Input: dimensioned drawing with shaded views. Units: mm. Origin: part minimum x, y, z. A direction names the side the tool comes from. Give positions to 0.01 mm unless a question says otherwise; leave off trailing zeros. Write each loop counter-clockwise with the first axis right and the second up, starting at its lowest first coordinate (ties: lowest second). Pieces come first, ordered by that corner, then holes. Notation, with made-up numbers: (28.25, 22.5) -> (54.25, 22.5) arc R6 cw to (54.25, 26.5) -> close; hole circle Ø4 at (-39, 55). An arc over 180 degrees is marked (long way). Answer as a JSON object with one key per item and string values.
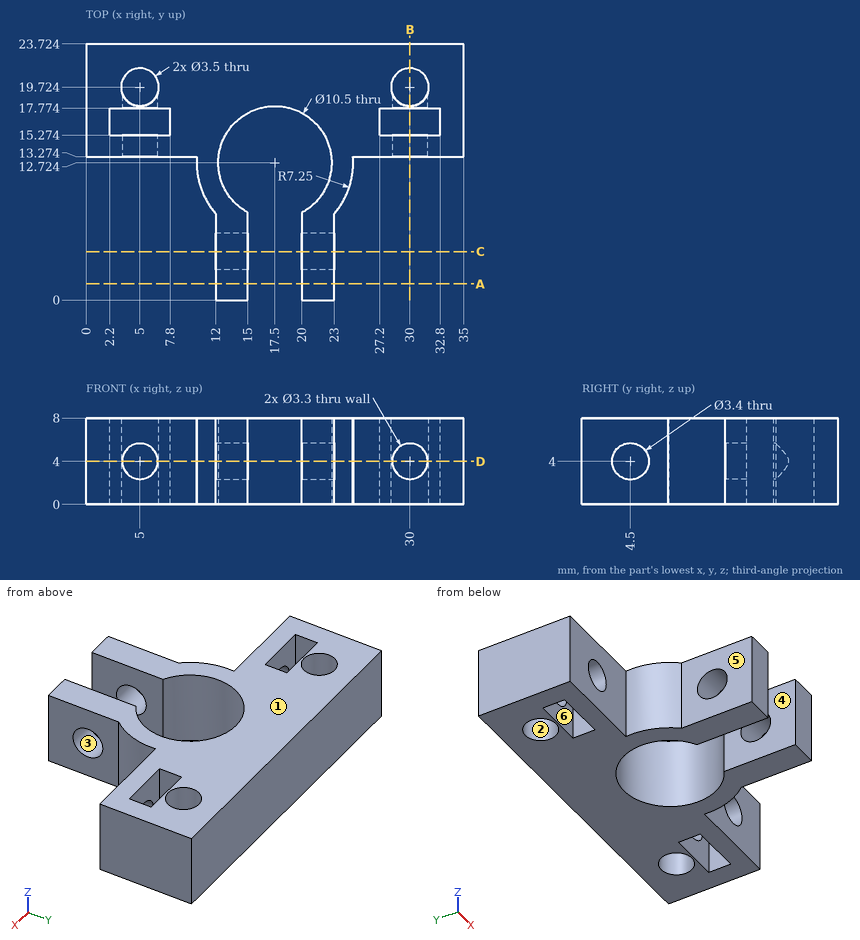
Q1. Cut plane B-B (x = 30). Return the cut outline in (y, z).
Values:
{"outline": "(13.27, 0) -> (15.27, 0) -> (15.27, 2.35) -> (13.27, 2.35) -> close; (13.27, 5.65) -> (15.27, 5.65) -> (15.27, 8) -> (13.27, 8) -> close; (17.77, 0) -> (17.97, 0) -> (17.97, 2.35) -> (17.77, 2.35) -> close; (17.77, 5.65) -> (17.97, 5.65) -> (17.97, 8) -> (17.77, 8) -> close; (21.47, 0) -> (23.72, 0) -> (23.72, 8) -> (21.47, 8) -> close"}
Q2. Cut plane C-C (y = 4.5). Return the cut outline in (x, z), and give its area (3 significant figures).
Values:
{"outline": "(12, 0) -> (15, 0) -> (15, 2.3) -> (12, 2.3) -> close; (12, 5.7) -> (15, 5.7) -> (15, 8) -> (12, 8) -> close; (20, 0) -> (23, 0) -> (23, 2.3) -> (20, 2.3) -> close; (20, 5.7) -> (23, 5.7) -> (23, 8) -> (20, 8) -> close", "area": "27.6 mm²"}
Q3. Mould query, pull axis Z, two halves, no side actions, for the marked faces 1, 2 and 3. Classes: pulls with the +Z half, pulls with the -Z half, needs draft (parallel to the pull), parting line crosses it, or undercut.
Values:
{"face 1": "pulls with the +Z half", "face 2": "needs draft", "face 3": "undercut"}
Q4. Cut plane A-A (y = 1.5). Return the cut outline in (x, z).
Values:
{"outline": "(12, 0) -> (15, 0) -> (15, 8) -> (12, 8) -> close; (20, 0) -> (23, 0) -> (23, 8) -> (20, 8) -> close"}
Q5. First-contact query: P1, Ø1.5, axis at x = 26.5, z = 5.5, coming from the -Y side; P2, Ø2, axis at x = 30, z = 4, coming from the -Y side; P3, Ø2, axis at y = 12, z = 1, coming from the +X side. Flat tips, straight axial feed; report the tip coordinate or a pass-through.
Values:
{"P1": "y = 13.27", "P2": "y = 21.16", "P3": "x = 24.75"}
Q6. Material intervals for L1, parallel to X at y = 7.25, z = 6; L2, parallel to X at y = 14.5, z = 2.5 (1 decimal); L3, parallel to X at y = 17, z = 2 (1 decimal), sorted ascending. Write a range as from..to.
Values:
{"L1": "12..15, 20..23", "L2": "0..4.3, 5.7..12.6, 22.4..29.3, 30.7..35", "L3": "0..2.2, 7.8..14.5, 20.5..27.2, 32.8..35"}
Q7. Cut plane D-D (z = 4). State how many separate pieces and enclosed holes the cut face has, and give its area (3 significant figures).
Values:
{"separate pieces": "3", "enclosed holes": "0", "area": "316 mm²"}
Q8. Set-up query: the marked faces 4, 5 and 6. Return all of +Z, -Z, +X, -X, +Y, -Y with unobstructed straight access to the full face (end or side cutting, diameter ignored); none if empty.
Values:
{"face 4": "+Z, -Z, -Y", "face 5": "+Z, -Z, -X, -Y", "face 6": "+Z, -Z"}
